```python
from build123d import *

# Parameters (mm, degrees)
ESQUISSE1_W             = 5
ESQUISSE1_H             = 30
ESQUISSE1_W_2           = 8.5
ESQUISSE1_H_2           = 10
BOSS_EXTRU_1_DEPTH      = 8.5
ESQUISSE2_R             = 1.8
ENL_V_MAT_EXTRU_1_DEPTH = 20
CONG_3_R                = 3
CONG_1_R                = 2


with BuildPart() as part:
    # Esquisse1 → Boss.-Extru.1 (new body)
    with BuildSketch(Plane.XY):
        with Locations((2.5, 15)):
            Rectangle(ESQUISSE1_W, ESQUISSE1_H)
        with Locations((16, 15)):
            Rectangle(ESQUISSE1_W, ESQUISSE1_H)
        with Locations((9.25, 15)):
            Rectangle(ESQUISSE1_W_2, ESQUISSE1_H_2)
    extrude(amount=BOSS_EXTRU_1_DEPTH)

    # Esquisse2 → Enlèv. mat.-Extru.1 (cut)
    with BuildSketch(Plane(origin=(18.5, 0, 0), x_dir=(0, 0, -1), z_dir=(1, 0, 0))):
        with Locations(Location((-4.25, 25, 0), (0, 0, 90))):
            Circle(ESQUISSE2_R)
        with Locations(Location((-4.25, 5, 0), (0, 0, 90))):
            Circle(ESQUISSE2_R)
    extrude(amount=-ENL_V_MAT_EXTRU_1_DEPTH, mode=Mode.SUBTRACT)

    # Congé3
    cong_3_edges = [part.edges().sort_by_distance(p)[0] for p in [
        (2.5, 30, 8.5),
        (9.25, 20, 0),
        (16, 30, 0),
        (16, 0, 0),
        (9.25, 10, 0),
        (2.5, 0, 0),
        (2.5, 30, 0),
        (2.5, 0, 8.5),
        (9.25, 10, 8.5),
        (16, 0, 8.5),
        (16, 30, 8.5),
        (9.25, 20, 8.5),
    ]]
    fillet(cong_3_edges, radius=CONG_3_R)

    # Congé1
    # the kernel refuses this fillet: 2 mm, written as the material it adds along each edge
    with BuildSketch(Plane(origin=(13.5, 10, 3), x_dir=(0, -1, 0), z_dir=(0, 0, 1)), Plane(origin=(5, 20, 3), x_dir=(0, 1, 0), z_dir=(0, 0, 1))) as cong_1_piece_1:
        with BuildLine():
            CenterArc((CONG_1_R, -CONG_1_R), CONG_1_R, 90, 90)
            Line((0, -CONG_1_R), (0, 0))
            Line((0, 0), (CONG_1_R, 0))
        make_face()
    extrude(amount=2.5)
    with BuildSketch(Plane(origin=(13.5, 17, 3), x_dir=(0, -0.9953436464450918, 0.09638996566753391), z_dir=(0, 0.09638996566753391, 0.9953436464450918))) as cong_1_piece_2_section:
        with BuildLine():
            CenterArc((3 + CONG_1_R, -CONG_1_R), CONG_1_R, 90, 90)
            Line((3, -CONG_1_R), (3, 0))
            Line((3, 0), (3 + CONG_1_R, 0))
        make_face()
    cong_1_piece_2 = revolve(axis=Axis((13.5, 17, 3), (1, 0, 0)), revolution_arc=185.531326158, mode=Mode.PRIVATE)
    cong_1_piece_2 = split(cong_1_piece_2, bisect_by=Plane(origin=(12.926399559, 19.220886719, 0), z_dir=(0, 0, 1)), keep=Keep.TOP, mode=Mode.PRIVATE)
    add(cong_1_piece_2)
    with BuildSketch(Plane(origin=(5, 17, 3), x_dir=(0, -0.9953436464450918, 0.09638996566753227), z_dir=(0, 0.09638996566753227, 0.9953436464450918))) as cong_1_piece_3_section:
        with BuildLine():
            CenterArc((3 + CONG_1_R, CONG_1_R), CONG_1_R, 180, 90)
            Line((3 + CONG_1_R, 0), (3, 0))
            Line((3, 0), (3, CONG_1_R))
        make_face()
    cong_1_piece_3 = revolve(axis=Axis((5, 17, 3), (1, 0, 0)), revolution_arc=185.531326158, mode=Mode.PRIVATE)
    cong_1_piece_3 = split(cong_1_piece_3, bisect_by=Plane(origin=(5.573600437, 19.220886663, 0), z_dir=(0, 0, 1)), keep=Keep.TOP, mode=Mode.PRIVATE)
    add(cong_1_piece_3)
    with BuildSketch(Plane(origin=(13.5, 13, 3), x_dir=(0, 0.9953436464450918, 0.09638996566753272), z_dir=(0, -0.09638996566753272, 0.9953436464450918))) as cong_1_piece_4_section:
        with BuildLine():
            CenterArc((3 + CONG_1_R, CONG_1_R), CONG_1_R, 180, 90)
            Line((3 + CONG_1_R, 0), (3, 0))
            Line((3, 0), (3, CONG_1_R))
        make_face()
    cong_1_piece_4 = revolve(axis=Axis((13.5, 13, 3), (-1, 0, 0)), revolution_arc=185.531326158, mode=Mode.PRIVATE)
    cong_1_piece_4 = split(cong_1_piece_4, bisect_by=Plane(origin=(12.926399561, 10.779113284, 0), z_dir=(0, 0, 1)), keep=Keep.TOP, mode=Mode.PRIVATE)
    add(cong_1_piece_4)
    with BuildSketch(Plane(origin=(5, 13, 3), x_dir=(0, 0.9953436464450918, 0.09638996566753391), z_dir=(0, -0.09638996566753391, 0.9953436464450918))) as cong_1_piece_5_section:
        with BuildLine():
            CenterArc((3 + CONG_1_R, -CONG_1_R), CONG_1_R, 90, 90)
            Line((3, -CONG_1_R), (3, 0))
            Line((3, 0), (3 + CONG_1_R, 0))
        make_face()
    cong_1_piece_5 = revolve(axis=Axis((5, 13, 3), (-1, 0, 0)), revolution_arc=185.531326158, mode=Mode.PRIVATE)
    cong_1_piece_5 = split(cong_1_piece_5, bisect_by=Plane(origin=(5.573600429, 10.779113281, 0), z_dir=(0, 0, 1)), keep=Keep.TOP, mode=Mode.PRIVATE)
    add(cong_1_piece_5)
    with BuildSketch(Plane(origin=(13.5, 17, 5.5), x_dir=(0, -0.9953436464450917, -0.09638996566753434), z_dir=(0, 0.09638996566753434, -0.9953436464450917))) as cong_1_piece_6_section:
        with BuildLine():
            CenterArc((3 + CONG_1_R, CONG_1_R), CONG_1_R, 180, 90)
            Line((3, CONG_1_R), (3, 0))
            Line((3, 0), (3 + CONG_1_R, 0))
        make_face()
    cong_1_piece_6 = revolve(axis=Axis((13.5, 17, 5.5), (-1, 0, 0)), revolution_arc=185.531326158, mode=Mode.PRIVATE)
    cong_1_piece_6 = split(cong_1_piece_6, bisect_by=Plane(origin=(12.92639966, 19.220886752, 8.5), z_dir=(0, 0, -1)), keep=Keep.TOP, mode=Mode.PRIVATE)
    add(cong_1_piece_6)
    with BuildSketch(Plane(origin=(5, 17, 5.5), x_dir=(0, -0.9953436464450918, -0.09638996566753258), z_dir=(0, 0.09638996566753258, -0.9953436464450918))) as cong_1_piece_7_section:
        with BuildLine():
            CenterArc((3 + CONG_1_R, -CONG_1_R), CONG_1_R, 90, 90)
            Line((3, -CONG_1_R), (3, 0))
            Line((3, 0), (3 + CONG_1_R, 0))
        make_face()
    cong_1_piece_7 = revolve(axis=Axis((5, 17, 5.5), (-1, 0, 0)), revolution_arc=185.531326158, mode=Mode.PRIVATE)
    cong_1_piece_7 = split(cong_1_piece_7, bisect_by=Plane(origin=(5.573251137, 19.22118781, 8.5), z_dir=(0, 0, -1)), keep=Keep.TOP, mode=Mode.PRIVATE)
    add(cong_1_piece_7)
    with BuildSketch(Plane(origin=(13.5, 13, 5.5), x_dir=(0, 0.9953436464450918, -0.09638996566753316), z_dir=(0, -0.09638996566753316, -0.9953436464450918))) as cong_1_piece_8_section:
        with BuildLine():
            CenterArc((3 + CONG_1_R, -CONG_1_R), CONG_1_R, 90, 90)
            Line((3, -CONG_1_R), (3, 0))
            Line((3, 0), (3 + CONG_1_R, 0))
        make_face()
    cong_1_piece_8 = revolve(axis=Axis((13.5, 13, 5.5), (1, 0, 0)), revolution_arc=185.531326158, mode=Mode.PRIVATE)
    cong_1_piece_8 = split(cong_1_piece_8, bisect_by=Plane(origin=(12.926652362, 10.77922389, 8.5), z_dir=(0, 0, -1)), keep=Keep.TOP, mode=Mode.PRIVATE)
    add(cong_1_piece_8)
    with BuildSketch(Plane(origin=(5, 13, 5.5), x_dir=(0, 0.9953436464450917, -0.09638996566753434), z_dir=(0, -0.09638996566753434, -0.9953436464450917))) as cong_1_piece_9_section:
        with BuildLine():
            CenterArc((3 + CONG_1_R, CONG_1_R), CONG_1_R, 180, 90)
            Line((3, CONG_1_R), (3, 0))
            Line((3, 0), (3 + CONG_1_R, 0))
        make_face()
    cong_1_piece_9 = revolve(axis=Axis((5, 13, 5.5), (1, 0, 0)), revolution_arc=185.531326158, mode=Mode.PRIVATE)
    cong_1_piece_9 = split(cong_1_piece_9, bisect_by=Plane(origin=(5.573600352, 10.779113305, 8.5), z_dir=(0, 0, -1)), keep=Keep.TOP, mode=Mode.PRIVATE)
    add(cong_1_piece_9)
    with BuildSketch(Plane(origin=(13.5, 20, 3), x_dir=(0, 1, 0), z_dir=(0, 0, 1)), Plane(origin=(5, 10, 3), x_dir=(0, -1, 0), z_dir=(0, 0, 1))) as cong_1_piece_10:
        with BuildLine():
            CenterArc((CONG_1_R, CONG_1_R), CONG_1_R, 180, 90)
            Line((0, CONG_1_R), (0, 0))
            Line((0, 0), (CONG_1_R, 0))
        make_face()
    extrude(amount=2.5)


solid = part.part
```
Can you work these out from the model? Positions are in its coordinate system, mm. A direction names the side the tool comes from. Give positions to 0.01 mm unless a question says otherwise; leave off trailing zeros. Loops run counter-clockwise (first coordinate to the right, second up) from the corner with the lowest first, then second, coordinate; pieces in that order, holes last. Notation, with made-up numbers: M -12.75,-22 L 12.25,-22 A7 cw 12.25,-12 Z; hole C 40,39.5 d7. An arc over 180 degrees is marked long. One line per item, written item: value.
(1) Suppose I cut it at A-A on x = 15. List the corners of the cut face in (y, z) for me.
Returned:
outline: M 0,3 A3 ccw 3,0 L 27,0 A3 ccw 30,3 L 30,5.5 A3 ccw 27,8.5 L 3,8.5 A3 ccw 0,5.5 Z; hole C 5,4.25 d3.6; hole C 25,4.25 d3.6
(2) Suppose I cut it at C-C on y = 5. List the corners of the cut face in (x, z) for me, plus the area to 3 significant figures.
Returned:
outline: M 0,0 L 5,0 L 5,2.45 L 0,2.45 Z; M 0,6.05 L 5,6.05 L 5,8.5 L 0,8.5 Z; M 13.5,0 L 18.5,0 L 18.5,2.45 L 13.5,2.45 Z; M 13.5,6.05 L 18.5,6.05 L 18.5,8.5 L 13.5,8.5 Z
area: 49.0 mm^2
(3) Suppose I cut it at D-D on x = 9.25. List the corners of the cut face in (y, z) for me, plus the area to 3 significant figures.
Returned:
outline: M 10,3 A3 ccw 13,0 L 17,0 A3 ccw 20,3 L 20,5.5 A3 ccw 17,8.5 L 13,8.5 A3 ccw 10,5.5 Z
area: 77.3 mm^2
(4) Suppose I cut it at B-B on z = 4.25. Count the separate pieces of the cut face and the enclosed holes in it, plus the area to 3 significant figures.
Returned:
separate pieces: 5
enclosed holes: 0
area: 316 mm^2
(5) Will these pins go through, and if not, where does the flat tip stop? pin 1 (1 mm diameter, centred on x = 12, z = 5, fed in from +Y); pin 2 (2 mm diameter, centred on x = 9, z = 3.5, fed in from -Y); pin 3 (0.8 mm diameter, centred on x = 9, z = 4, fed in from +Y).
Returned:
pin 1: y = 20.27
pin 2: y = 10
pin 3: y = 20
(6) We'd pull the mould along X, two halves only. Please class faces 4 (the face through (0, 15, 4)), 5 (the face through (2.54, 29.1, 0.86)), 6 (the face through (5, 3, 3)), 7 (the face through (9.28, 19.1, 0.86)): released by +X, released by -X, zero draft, split by the parting line, or undercut.
Returned:
face 4: released by -X
face 5: zero draft
face 6: undercut
face 7: undercut
(7) Which directions (+Z, -Z, +X, -X, +Y, -Y) give clear straight access to the entire face, cutting with the end or side of a thin tool? Please do faces 1 (the face through (16, 0, 4)), 2 (the face through (12.9, 20.57, 4.23)), 3 (the face through (9.28, 10.9, 0.86)).
Returned:
face 1: +Z, -Z, +X, -X, -Y
face 2: +Z, -Z, +Y
face 3: -Z, -Y
(8) I need wall thicknesses on line 1 (X direction, y = 26.75, z = 1.5); line 2 (Y direction, x = 4, z = 5); line 3 (Y direction, x = 2.5, z = 4). Which ranges of each line are inside material? Lowest first, please.
Returned:
line 1: 0 to 5, 13.5 to 18.5
line 2: 0 to 3.36, 6.64 to 23.36, 26.64 to 30
line 3: 0 to 3.22, 6.78 to 23.22, 26.78 to 30
